Can you work these out from the drawing? Everything is in mm from the part's minimum corner. Round coordinates to 2 decimals unless told otherwise and drop trailing zeros. Write each loop counter-clockwise with the first axis right and the second up, starting at its lowest first coordinate (ties: lowest second). Pieces come first, ordered by that corner, then holes. Notation, with made-up numbers: (73, 85) -> (86, 85) arc R15 ccw to (86, 90) -> close; hole circle Ø7 at (-16.5, -1.5). An arc over 180 degrees is marked (long way). Answer as CSV lines item,"result".
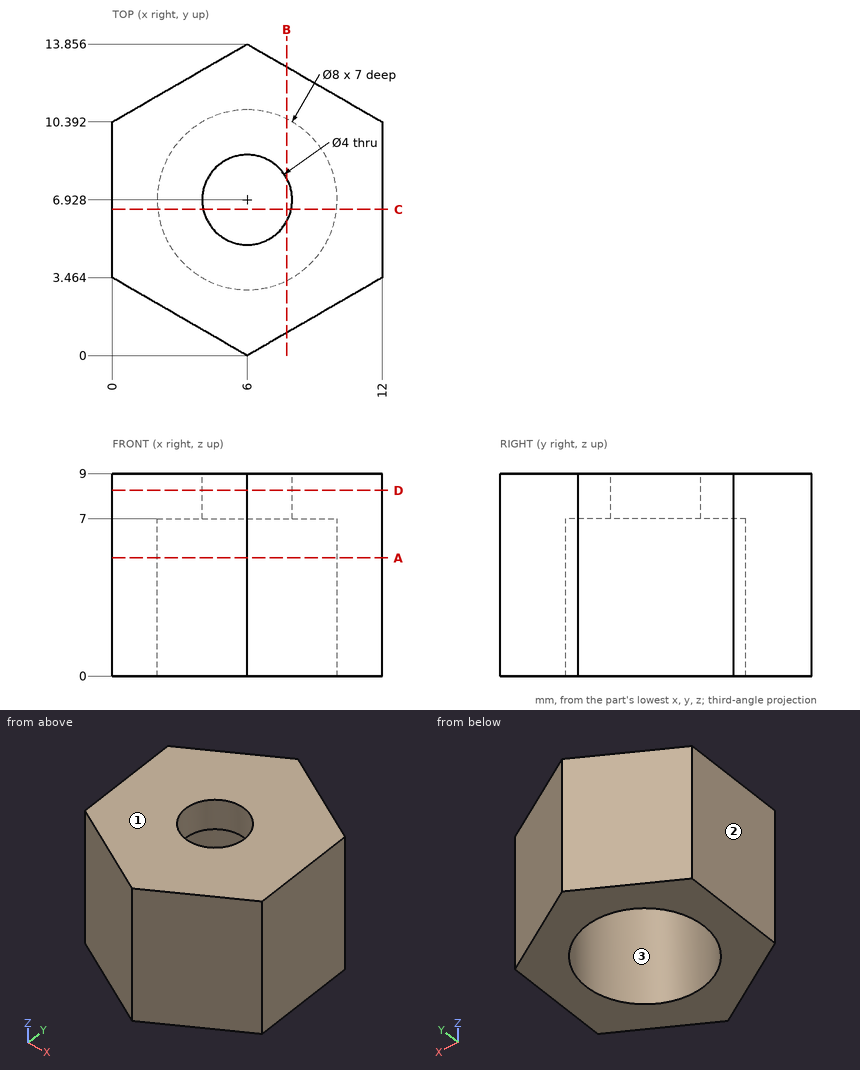
Item 1: Suppose I cut it at C-C, the plane y = 6.5. List the corners of the cut face in (x, z) for me.
Results found:
outline,"(0, 0) -> (2.02, 0) -> (2.02, 7) -> (4.05, 7) -> (4.05, 9) -> (0, 9) -> close; (7.95, 7) -> (9.98, 7) -> (9.98, 0) -> (12, 0) -> (12, 9) -> (7.95, 9) -> close"
Item 2: Suppose I cut it at D-D, the plane z = 8.25. List the corners of the cut face in (x, y) for me, then the cut area to 3 significant figures.
Results found:
outline,"(0, 3.46) -> (6, 0) -> (12, 3.46) -> (12, 10.39) -> (6, 13.86) -> (0, 10.39) -> close; hole circle Ø4 at (6, 6.93)"
area,"112 mm²"
Item 3: If we mould it in two halves opening along X, with no side actions, what happens to the marked faces 1, 2 and 3? For each: pulls with the +X half, pulls with the -X half, needs draft (parallel to the pull), parting line crosses it, or undercut.
Results found:
face 1,"needs draft"
face 2,"pulls with the -X half"
face 3,"undercut"
Item 4: Will this pin go through, and if not, where does the flat tip stop? pin 1 (2.5 mm diameter, centred on x = 6, y = 6.93, fed in from +Z).
Results found:
pin 1,"passes through"
Item 5: I need wall thicknesses on L1, parallel to X at y = 4.25, z = 2; L2, parallel to X at y = 7.5, z = 6; L3, parallel to Z at x = 4, y = 10.25. Which ranges of each line are inside material? Lowest first, please.
Results found:
L1,"x = 0 to 3.03, 8.97 to 12"
L2,"x = 0 to 2.04, 9.96 to 12"
L3,"z = 7 to 9"
Item 6: Suppose I cut it at B-B, the plane x = 7.75. List the corners of the cut face in (y, z) for me (1 decimal).
Results found:
outline,"(1, 0) -> (3.3, 0) -> (3.3, 7) -> (6, 7) -> (6, 9) -> (1, 9) -> close; (7.9, 7) -> (10.5, 7) -> (10.5, 0) -> (12.8, 0) -> (12.8, 9) -> (7.9, 9) -> close"
Item 7: Suppose I cut it at A-A, the plane z = 5.25. List the corners of the cut face in (x, y) for me.
Results found:
outline,"(0, 3.46) -> (6, 0) -> (12, 3.46) -> (12, 10.39) -> (6, 13.86) -> (0, 10.39) -> close; hole circle Ø8 at (6, 6.93)"
